```python
from build123d import *

# Parameters (mm, degrees)
SKETCH1_R           = 63.5
BOSS_EXTRUDE2_DEPTH = 12.7
FILLET2_R           = 3.17
CUT_EXTRUDE1_DEPTH  = 13.7


with BuildPart() as part:
    # Sketch1 → Boss-Extrude2 (new body)
    with BuildSketch(Plane(origin=(0, 0, 0), x_dir=(1, 0, 0), z_dir=(0, 1, 0))):
        Circle(SKETCH1_R)
    extrude(amount=BOSS_EXTRUDE2_DEPTH)

    # Fillet2
    fillet2_edges = [part.edges().sort_by_distance(p)[0] for p in [
        (-63.5, 12.7, 0),
    ]]
    fillet(fillet2_edges, radius=FILLET2_R)

    # Sketch3 → Cut-Extrude1 (cut, through all)
    with BuildSketch(Plane(origin=(0, 12.7, 0), x_dir=(1, 0, 0), z_dir=(0, 1, 0))):
        with BuildLine():
            Line((-50.8, 7.49), (-63.056719705, 7.49))
            ThreePointArc((-63.056719705, 7.49), (-63.5, 0), (-63.056719705, -7.49))
            Line((-63.056719705, -7.49), (-50.8, -7.49))
            ThreePointArc((-50.8, -7.49), (-43.31, 0), (-50.8, 7.49))
        make_face()
        with BuildLine():
            Line((50.8, -7.49), (63.056719705, -7.49))
            ThreePointArc((63.056719705, -7.49), (63.5, 0), (63.056719705, 7.49))
            Line((63.056719705, 7.49), (50.8, 7.49))
            ThreePointArc((50.8, 7.49), (43.31, 0), (50.8, -7.49))
        make_face()
    extrude(amount=-CUT_EXTRUDE1_DEPTH, mode=Mode.SUBTRACT)


solid = part.part
```
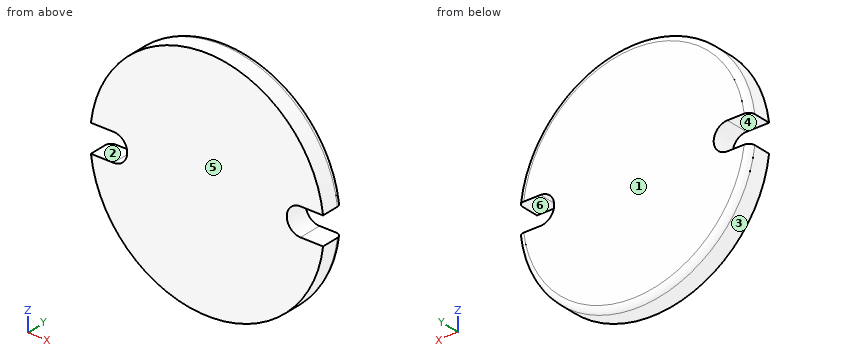
Work out the finished part from the listing and answer in its coordinate system (mm). Face numbers are marked on the shaded views. A direction names the side the tool comes from. Coordinates: 2 decimals unless noted, no trailing zeros. Loops run counter-clockwise (first coordinate to the right, second up) from the corner with the lowest first, then second, coordinate; pieces in that order, holes last. Notation, with made-up numbers: M 16,77 L 42,77 A19 cw 42,114 Z; hole C 2,81.5 d4. An arc over 180 degrees is marked long. Use CSV: the item, a comma, the result in double quotes. Start each with the question number.
(1) Given pin 1 Ø6 at (x, y) = (56, 5.5) entering from -Z (3 decimals); pin 2 Ø5 at (y, z) = (7, 41) entering from +X; pin 3 Ø1.5 at (y, z) = (2, -46.5) entering from +X; pin 4 Ø4 at (x, z) = (-27.5, -9.5) entering from -Y, each flat-ended and moving along its own axis, determine where each tip first touches the part or whether it passes through.
(2) Find section A-A, the plane y = 7. Give the vertices of the cut face in (x, z).
(3) For the marked faces 4, 5 and 6, determine the directions among +Z, -Z, +X, -X, +Y, -Y from which every point of the face is accessible in a straight line to the end or side of a thin tool.
(4) Find section B-B, the plane z = 0. Give the vertices of the cut face in (x, y).
(5) For a pull along Z with two mould halves and no side action, classify the marked faces 1, 2 and 3 as +Z half, -Z half, draft (parallel to the pull), parting line (faces both ways), or undercut.
(6) Consider line 1 (Y direction, x = 29, z = -53); line 2 (Z direction, x = -56, y = 11); line 3 (Z direction, x = -47.5, y = 4). Determine where each line is inside the solid, lowest interval first.
Recorded:
1,pin 1,"stops at z = -34.975"
1,pin 2,"stops at x = 50.5"
1,pin 3,"stops at x = 44.04"
1,pin 4,"stops at y = 0"
2,outline,"M -63.06,-7.49 A63.5 ccw 63.06,-7.49 L 50.8,-7.49 A7.49 cw 50.8,7.49 L 63.06,7.49 A63.5 ccw -63.06,7.49 L -50.8,7.49 A7.49 cw -50.8,-7.49 Z"
3,face 4,"-X, +Y, -Y"
3,face 5,"+Z, -Z, +X, -X, -Y"
3,face 6,"+X, +Y, -Y"
4,outline,"M -43.31,0 L 43.31,0 L 43.31,12.7 L -43.31,12.7 Z"
5,face 1,"draft"
5,face 2,"undercut"
5,face 3,"-Z half"
6,line 1,"y = 0 to 12.7"
6,line 2,"z = -29.16 to -7.49, 7.49 to 29.16"
6,line 3,"z = -42.14 to -6.72, 6.72 to 42.14"
